Could you check a few things on this model? Use its own coordinates, in mm. Face numbers are marked on the shaded views. Coordinates: 2 decimals unless noted, no trailing zeros. Write each loop counter-clockwise with the first axis right and the second up, starting at its lowest first coordinate (ties: lowest second). Pieces come first, ordered by that corner, then holes. Notation, with made-up numbers: (-34, -30) - (-4, -30) arc R15 ccw to (-4, -4) - close; hole circle Ø4 at (47, 23). An arc over 180 degrees is marked (long way). Answer as a JSON object with one key per item and string values. Group by question number.
1) If we section it at A-A (y = 393): Write out the boundary of the cut face in (x, z).
2) Please list where these lines run through material, in increasing order: line 1 along X through (y, z) = (868, 43.5); line 2 along Z through (x, y) = (157, 851).
3) If we section it at B-B (z = 42.5): Write out the boundary of the cut face in (x, y), plus the area to 3 significant figures.
4) We'd pull the mould along Y, two halves only. Please class the marked faces 1 and 2: released by +Y, released by -Y, zero draft, split by the parting line, or undercut.
```python
from build123d import *

# Parameters (mm, degrees)
F0_W     = 1000
F0_H     = 1000
F1_DEPTH = 50
F2_T     = -25
F3_R     = 12.5


with BuildPart() as f1:
    # F0 (on Top) → F1 (new body)
    with BuildSketch(Plane.XY):
        with Locations((500, 500)):
            Rectangle(F0_W, F0_H)
    extrude(amount=F1_DEPTH)

    # F2
    f2_openings = [f1.faces().sort_by_distance(p)[0] for p in [
        (500, 500, 50),
    ]]
    offset(amount=F2_T, openings=f2_openings)

    # F3
    f3_edges = [f1.edges().sort_by_distance(p)[0] for p in [
        (25, 975, 37.5),
        (975, 975, 37.5),
        (975, 25, 37.5),
        (25, 25, 37.5),
    ]]
    fillet(f3_edges, radius=F3_R)


solid = f1.part
```
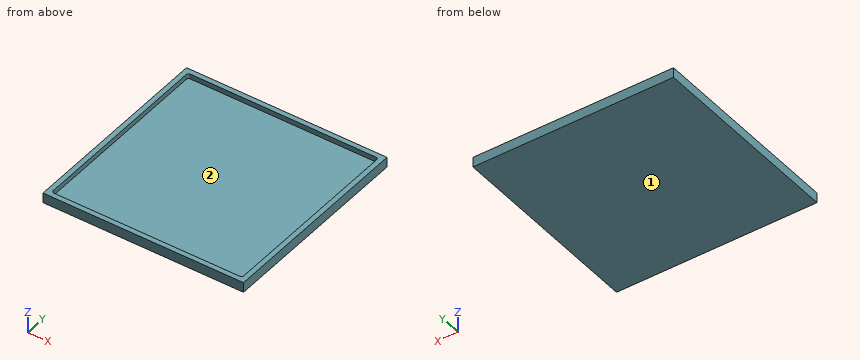
Here are the results:
{
 "1": {"outline": "(0, 0) - (1000, 0) - (1000, 50) - (975, 50) - (975, 25) - (25, 25) - (25, 50) - (0, 50) - close"},
 "2": {"line 1": "x = 0 to 25, 975 to 1000", "line 2": "z = 0 to 25"},
 "3": {"outline": "(0, 0) - (1000, 0) - (1000, 1000) - (0, 1000) - close; hole (25, 37.5) arc R12.5 ccw to (37.5, 25) - (962.5, 25) arc R12.5 ccw to (975, 37.5) - (975, 962.5) arc R12.5 ccw to (962.5, 975) - (37.5, 975) arc R12.5 ccw to (25, 962.5) - close", "area": "97,600 mm²"},
 "4": {"face 1": "zero draft", "face 2": "undercut"}
}
